The figure shows three views and two pictorial views of one solid part (mm, origin at its lowest corner). Answer the questions. Round coordinates to 2 decimals unless told otherwise and drop trailing zeros. Order: outer loops, then holes, each group sorted by start corner. A loop starts at its lowest first (then second) coordinate and runs counter-clockwise, first axis right, second up. Notation, with made-up numbers: M 23,85 L 63,85 A14 ccw 63,110 Z; hole C -26.5,-17.75 d1. An arc over 180 degrees is marked long. Return JSON: item names as keys, results as strings.
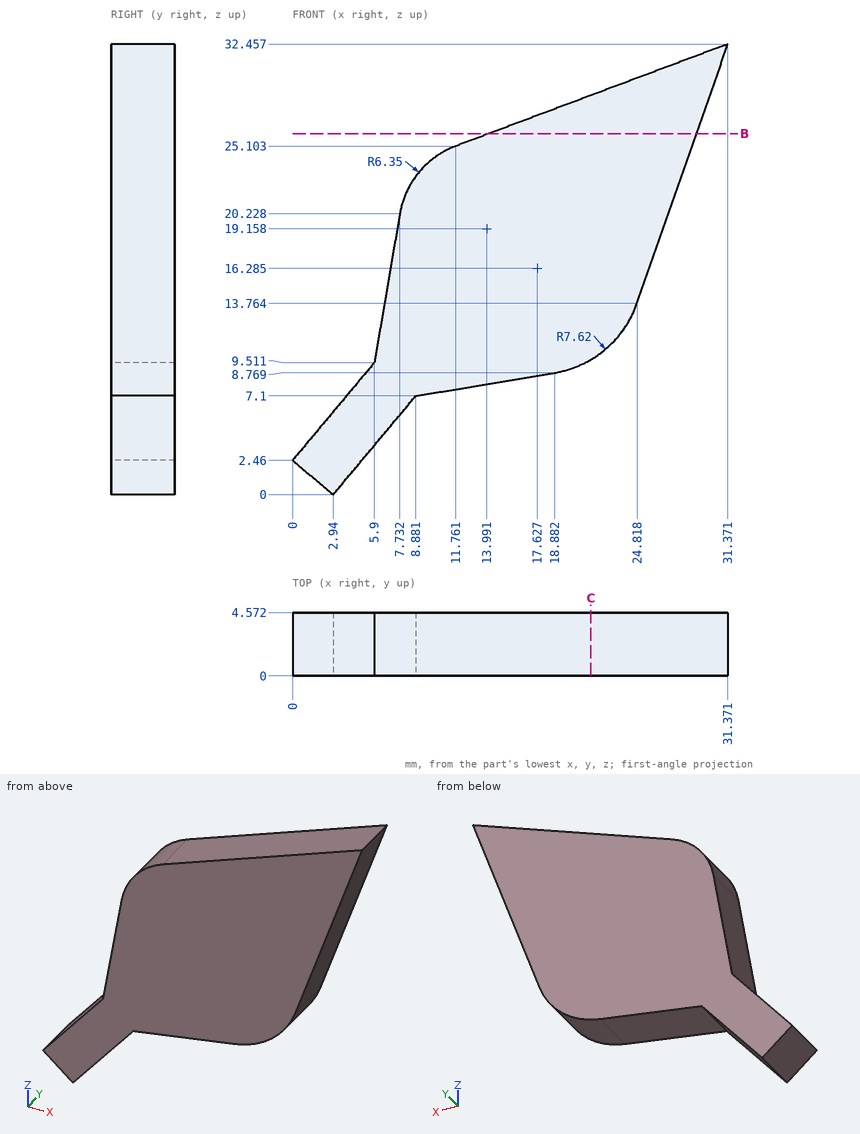
Item 1: Consider line 1 along X through (y, z) = (2.1, 24) (1 decimal); line 2 along X through (y, z) = (2.55, 3.5); line 3 along Z through (x, y) = (24, 0.4) (1 decimal). Determine where each line is inside the solid, lowest interval first. Write a range as [from, to].
Output:
{"line 1": "x = [9.9, 28.4]", "line 2": "x = [0.87, 5.87]", "line 3": "z = [12.1, 29.7]"}
Item 2: Find section C-C (x = 21.5). Determine the outline of the cut face in (y, z) (1 decimal).
Output:
{"outline": "M 0,9.7 L 4.6,9.7 L 4.6,28.8 L 0,28.8 Z"}
Item 3: Each of these flat-tipped pins is pushed along its axis until it touches: pin 1 (1 mm diameter, centred on y = 3.5, z = 18, fed in from -X) (1 decimal); pin 2 (2 mm diameter, centred on x = 13, y = 3, fed in from -Z); pin 3 (4 mm diameter, centred on x = 16.5, z = 7.5, fed in from -Y). Where does it stop, or does it pass through?
Output:
{"pin 1": "stops at x = 7.3", "pin 2": "stops at z = 7.62", "pin 3": "stops at y = 0"}
Item 4: Find section B-B (z = 26). Determine the outline of the cut face in (x, y).
Output:
{"outline": "M 14.15,0 L 29.11,0 L 29.11,4.57 L 14.15,4.57 Z"}
